Could you check a few things on this drawing? It's one solid part, dimensions in mm from its lowest x, y, z. Round coordinates to 2 decimals unless told otherwise and drop trailing zeros. Loops run counter-clockwise (first coordinate to the right, second up) from the corner with the lowest first, then second, coordinate; pieces in that order, holes last. Notation, with made-up numbers: M 71.5,40.5 L 113.5,40.5 A6 ccw 113.5,47.5 Z; hole C 40,-38.75 d8. An arc over 180 degrees is marked long. Answer as CSV lines item,"result".
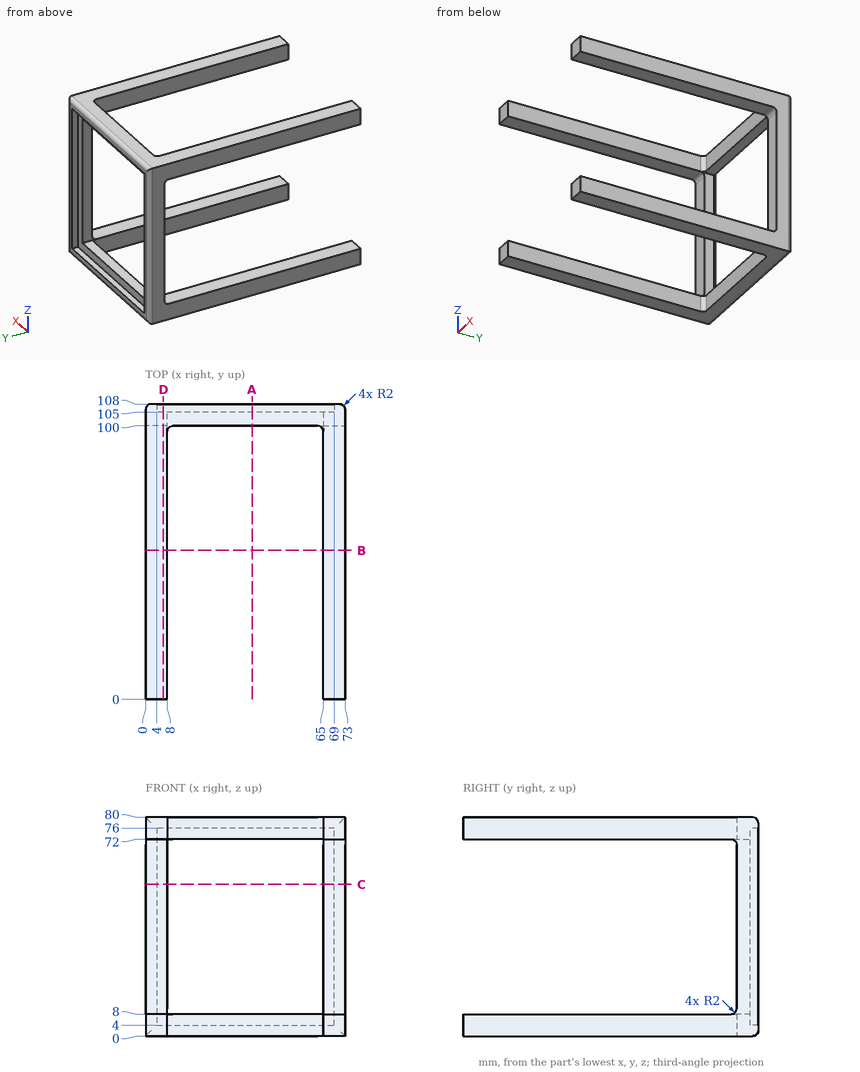
Item 1: Will these pins go through, and if not, where does the flat tip stop? pin 1 (4 mm diameter, centred on x = 69, z = 41.5, fed in from -Y); pin 2 (6 mm diameter, centred on y = 96, z = 19.5, fed in from -X); pin 3 (0.9 mm diameter, centred on x = 45, y = 107, fed in from -Z).
Output:
pin 1,"stops at y = 100"
pin 2,"passes through"
pin 3,"stops at z = 0.08"
Item 2: If we section it at C-C on z = 55.5: Write out the boundary of the cut face in (x, y).
Output:
outline,"M 0,100 L 8,100 L 8,105 L 4,105 L 4,108 L 2,108 A2 ccw 0,106 Z; M 65,100 L 73,100 L 73,106 A2 ccw 71,108 L 69,108 L 69,105 L 65,105 Z"
Item 3: If I drill on line 1 along X through (y, z) = (102, 48); line 2 along Z through (x, y) = (68, 39); line 3 along Y through (x, z) = (38, 76.5), over which ranges is the centre line in solid material (lowest first)? Write a range as from..to.
Output:
line 1,"x = 0..8, 65..73"
line 2,"z = 0..8, 72..80"
line 3,"y = 100..108"
Item 4: If we section it at A-A on x = 39: Write out the boundary of the cut face in (y, z), then the cut area to 3 significant figures.
Output:
outline,"M 100,0 L 106,0 A2 ccw 108,2 L 108,4 L 105,4 L 105,8 L 100,8 Z; M 100,72 L 105,72 L 105,76 L 108,76 L 108,78 A2 ccw 106,80 L 100,80 Z"
area,"102 mm2"
Item 5: If we section it at D-D on x = 6.5: Write out the boundary of the cut face in (y, z), then the cut area to 3 significant figures.
Output:
outline,"M 0,0 L 106,0 A2 ccw 108,2 L 108,4 L 105,4 L 105,76 L 108,76 L 108,78 A2 ccw 106,80 L 0,80 L 0,72 L 98,72 A2 cw 100,70 L 100,10 A2 cw 98,8 L 0,8 Z"
area,"2,020 mm2"
Item 6: If we section it at B-B on y = 54.5: Write out the boundary of the cut face in (x, z), then the cut area to 3 significant figures.
Output:
outline,"M 0,0 L 8,0 L 8,8 L 0,8 Z; M 0,72 L 8,72 L 8,80 L 0,80 Z; M 65,0 L 73,0 L 73,8 L 65,8 Z; M 65,72 L 73,72 L 73,80 L 65,80 Z"
area,"256 mm2"
